Model file for the job. Use its own axes, mm. A direction names the side the tool comes from. Give positions to 0.01 mm unless a question says otherwise; leave off trailing zeros. Write each loop counter-clockwise with the first axis right and the second up, starting at its lowest first coordinate (ties: lowest second). Pieces come first, ordered by that corner, then holes. Notation, with made-up numbers: (1, -11.5) - (6, -11.5) arc R26 cw to (6, 23.5) - close; hole circle Ø7 at (-37.5, 39.25). An arc over 180 degrees is marked (long way). Use CSV: the item, a comma, the result in double quotes.
Autodesk Inventor part; units mm, degrees
ref_plane "Work Plane1" through (-5.5, 5, -9) normal (0, 0, 1) x (1, 0, 0)
ref_plane "YZ Plane" through (0, 0, 0) normal (1, 0, 0) x (0, 1, 0)
ref_plane "XZ Plane" through (0, 0, 0) normal (0, 1, 0) x (-1, 0, 0)
sketch "Sketch1" plane through (0, 0, 0) normal (0, 1, 0) x (-1, 0, 0)
  line L0 (0, 0) -> (0, -10.6)
  line L1 (0, -10.6) -> (-4.5, -10.6)
  line L2 (-4.5, -10.6) -> (-4.5, -39.4)
  line L3 (-4.5, -39.4) -> (0, -39.4)
  line L4 (0, -39.4) -> (0, -50)
  line L5 (0, -50) -> (10, -50)
  line L6 (10, -50) -> (10, -48)
  line L7 (10, -48) -> (15.5, -48)
  line L8 (15.5, -48) -> (15.5, -40)
  line L9 (15.5, -40) -> (10, -40)
  line L10 (10, -40) -> (10, -10)
  line L11 (10, -10) -> (15.5, -10)
  line L12 (15.5, -10) -> (15.5, -2)
  line L13 (15.5, -2) -> (10, -2)
  line L14 (10, -2) -> (10, 0)
  line L15 (10, 0) -> (0, 0)
  line L16 (10.5, -3) -> (0.5, -3)
  line L17 (0.5, -3) -> (0.5, -9)
  line L18 (0.5, -9) -> (10.5, -9)
  line L19 (10.5, -9) -> (10.5, -3)
  line L20 (10.5, -41) -> (0.5, -41)
  line L21 (0.5, -41) -> (0.5, -47)
  line L22 (0.5, -47) -> (10.5, -47)
  line L23 (10.5, -47) -> (10.5, -41)
  dimension "d0" = 20
  dimension "d1" = 50
  dimension "d2" = 10.6
  dimension "d3" = 10.6
  dimension "d4" = 2
  dimension "d5" = 2
  dimension "d6" = 8
  dimension "d7" = 8
  dimension "d8" = 4.5
  dimension "d9" = 5.5
  dimension "d10" = 5.5
  dimension "d11" = 5.5
  dimension "d12" = 5.5
  dimension "d13" = 10
  dimension "d14" = 6
  dimension "d15" = 5
  dimension "d16" = 3
  dimension "d17" = 10
  dimension "d18" = 6
  dimension "d19" = 3
extrude "Extrusion1" add sketch "Sketch1" along normal blind 5
sketch "Sketch2" plane through (-10.5, 0, -9) normal (0, 0, 1) x (1, 0, 0)
  point P0 (10.5, 0)
ref_plane "Work Plane1" through (-5.5, 5, -9) normal (0, 0, 1) x (1, 0, 0)
sketch "Sketch4" plane through (-5.5, 5, -9) normal (0, 0, 1) x (1, 0, 0)
  line L0 (-5, -5) -> (5, -5)
  line L1 (5, -5) -> (-5, -5)
  line L2 (-5, -5) -> (5, -5)
  line L3 (5, -5) -> (-5, -5)
  line L4 (-4.5, -5) -> (5.5, -5)
  line L5 (-10, -5) -> (-4.5, -5)
  line L6 (-4.5, -5) -> (-10, -5)
  line L7 (-10, -5) -> (-4.5, -5)
  line L8 (-4.5, -5) -> (-10, -5)
  line L9 (5.5, -5) -> (-4.5, -5)
  line L10 (10, -5) -> (5.5, -5)
  line L11 (5.5, -5) -> (10, -5)
  line L12 (-5, 0) -> (5, 0)
  line L13 (5, 0) -> (-5, 0)
  line L14 (-5, 0) -> (5, 0)
  line L15 (5, 0) -> (-5, 0)
  line L16 (5.5, 0) -> (10, 0)
  line L17 (10, 0) -> (5.5, 0)
  line L18 (5.5, 0) -> (-4.5, 0)
  line L19 (-4.5, 0) -> (-10, 0)
  line L20 (-10, 0) -> (-4.5, 0)
  line L21 (-4.5, 0) -> (-10, 0)
  line L22 (-10, 0) -> (-4.5, 0)
  line L23 (-4.5, 0) -> (5.5, 0)
  line L24 (5, -5) -> (5, 0)
  line L25 (-5, -5) -> (-5, 0)
  line L26 (5.5, -5) -> (-4.5, -5)
  line L27 (-5, -5) -> (-5, 0) construction
  line L28 (-5, -5) -> (0, -5) construction
  line L29 (5, -5) -> (5, 0)
  line L30 (5, -5) -> (5, 0) construction
  line L31 (5, -5) -> (10, -5) construction
  line L32 (-5, 0) -> (-5, -5)
  line L33 (0, -5) -> (5, -5)
  line L34 (5, 0) -> (5, -5)
  line L35 (5.5, 0) -> (-4.5, 0)
  line L36 (-5, -5) -> (0, -5)
  line L37 (-5, -5) -> (-1, -5)
  line L38 (-1, -5) -> (-1, -4)
  line L39 (5, -5) -> (1, -5)
  line L40 (1, -5) -> (1, -4)
  line L41 (-5, -5) -> (-5, -4)
  line L42 (-5, -5) -> (-5, 0)
  line L43 (5, -5) -> (5, -4)
  arc A0 (5, 0) -> (1, -4) centre (5, -4) ccw
  arc A1 (-1, -4) -> (-5, 0) centre (-5, -4) ccw
  dimension "d26" = 90
  dimension "d28" = 90
  dimension "d48" = 4
  dimension "d49" = 1
  dimension "d50" = 4
  dimension "d51" = 1
  dimension "d52" = 4
extrude "Extrusion2" add sketch "Sketch4" along normal blind 6 contours L25 A1 L38 L0 | L40 A0 L24 L0
sketch "Sketch6" plane through (-10, 0, -48) normal (0, 0, -1) x (-1, 0, 0)
  circle A0 centre (3, 2.5) radius 1.4
  line L0 (0, 0) -> (5.5, 0)
  line L1 (5.5, 0) -> (5.5, 5)
  line L2 (0, 5) -> (5.5, 5)
  line L3 (0, 0) -> (0, 5)
  point P0 (-10, 0)
  dimension "d34" = 2.5
  dimension "d35" = 2.5
  dimension "d47" = 2.8
extrude "Extrusion4" cut sketch "Sketch6" against normal through all contours A0
sketch "Sketch7" plane through (4.5, 0, -39.4) normal (0, 0, -1) x (-1, 0, 0)
  circle A0 centre (2.5, 2.5) radius 1
  line L0 (0, 5) -> (4.5, 5)
  line L1 (0, 0) -> (0, 5)
  point P0 (4.5, 0)
  dimension "d38" = 2
  dimension "d39" = 2.5
  dimension "d40" = 2.5
extrude "Extrusion5" cut sketch "Sketch7" against normal through all
sketch "Sketch8" plane through (-10, 0, -10) normal (0, 0, -1) x (-1, 0, 0)
  point P0 (-10, 0)
sketch "Sketch12" plane through (-0.5, 0, -41) normal (0, 0, -1) x (-1, 0, 0)
  line L0 (6, 1) -> (6, 0)
  line L1 (4, 0) -> (6, 0)
  line L2 (4, 0) -> (4, 1)
  arc A0 (4, 1) -> (0, 5) centre (0, 1) ccw
  line L3 (10, 5) -> (0, 5)
  arc A1 (10, 5) -> (6, 1) centre (10, 1) ccw
  arc A2 (4, 1) -> (0, 5) centre (0, 1) ccw
  arc A3 (10, 5) -> (6, 1) centre (10, 1) ccw
  line L4 (4, 0) -> (6, 0)
  line L5 (6, 1) -> (6, 0)
  line L6 (6, 0) -> (10, 0)
  line L7 (15, 0) -> (9.5, 0)
  line L8 (10, 5) -> (10, 0)
  line L9 (10, 0) -> (6, 0)
  line L10 (9.5, 0) -> (-0.5, 0)
  line L11 (4, 0) -> (0, 0)
  arc A4 (4, 1) -> (0, 5) centre (0, 1) ccw
  line L12 (0, 0) -> (0, 5)
  line L13 (4, 0) -> (4, 1)
  line L14 (4, 0) -> (4, 1)
  dimension "d54" = 5
extrude "Extrusion6" add sketch "Sketch12" along normal blind 6 contours A1 L8 L6 L0 | L10 L12 A0 L2
fillet "Fillet5" radius 2.5 6 edges at (-15.5, 5, -6) (-15.5, 5, -44) (4.5, 5, -25) (-15.5, 0, -6) (4.5, 0, -25) (-15.5, 0, -44)
sketch "Sketch13" plane through (0, 5, 0) normal (0, 1, 0) x (1, 0, 0)
  line L0 (-10, 0) -> (0, 0)
  line L1 (0, 0) -> (-1, 0)
  line L2 (-1, 0) -> (-1, 10.5)
  line L3 (-1, 10.5) -> (0, 10.5)
  line L4 (0, 10.5) -> (0, 0)
  line L5 (0, 39.4) -> (0, 50)
  line L6 (0, 39.4) -> (-1, 39.4)
  line L7 (-1, 39.4) -> (-1, 50)
  line L8 (-1, 50) -> (0, 50)
  line L9 (0, 50) -> (0, 39.4)
  dimension "d58" = 1
extrude "Extrusion7" cut sketch "Sketch13" against normal through all
sketch "Sketch14" plane through (0, 0, 0) normal (0, -1, 0) x (1, 0, 0)
  point P0 (0, 0)
sketch "Sketch15" plane through (0, 5, 0) normal (0, 1, 0) x (1, 0, 0)
  line L0 (-9.5, 23) -> (-2, 23)
  line L1 (-2, 23) -> (-2, 27)
  line L2 (-2, 27) -> (-9.5, 27)
  line L3 (-9.5, 27) -> (-9.5, 23)
  line L4 (-10, 0) -> (-1, 0)
  line L5 (-1, 39.4) -> (-1, 41)
  point P0 (0, 0)
  dimension "d61" = 4
  dimension "d62" = 7.5
  dimension "d63" = 23
  dimension "d64" = 1
extrude "Extrusion8" add sketch "Sketch15" along normal blind 4
sketch "Sketch17" plane through (-9.5, 5, -23) normal (0, 0, 1) x (1, 0, 0)
  line L0 (8.5, 0) -> (-1, 0)
  line L1 (0, 0) -> (0, 4)
  line L2 (0, 0) -> (0, 4)
  line L3 (0, 4) -> (1, 4)
  line L4 (7.5, 4) -> (0, 4)
  line L5 (1, 4) -> (0, 0)
  line L6 (7.5, 4) -> (7.5, 0)
  line L7 (7.5, 0) -> (7.5, 4)
  line L8 (7.5, 4) -> (6.5, 4)
  line L9 (6.5, 4) -> (7.5, 0)
  point P0 (9.5, -5)
  dimension "d69" = 1
  dimension "d70" = 1
extrude "Extrusion9" cut sketch "Sketch17" against normal through all contours L9 L4 L6 | L1 L3 L5
fillet "Fillet6" radius 2 4 edges at (-9, 7, -23) (-2.5, 7, -23) (-2.5, 7, -27) (-9, 7, -27)
sketch "Sketch18" plane through (0, 0, 0) normal (0, -1, 0) x (1, 0, 0)
  line L0 (0, -10.5) -> (0, -10.6)
  line L1 (0, -10.5) -> (0, -10.6)
  line L2 (0, -10.6) -> (-1, -10.6)
  line L3 (-1, -9) -> (-1, -10.5)
  line L4 (-1, -10.6) -> (-1, -10.5)
  line L5 (-1, -10.5) -> (0, -10.5)
  point P0 (0, 0)
  dimension "d74" = 1
extrude "Extrusion10" cut sketch "Sketch18" against normal through all
properties part number "tracks"
(1) Saw through at B-B, the plane z = -5. Count the separate pieces of the cut face and the enclosed holes in it, then the cut area to 3 significant figures.
Checked values:
separate pieces,"2"
enclosed holes,"1"
area,"46.8 mm^2"
(2) Flat gauge pins, fed straight in: P1, Ø1.5, axis at x = 1.5, y = 3, coming from the -Z side; P2, Ø1.6, axis at y = 3, z = -49, coming from the -X side; P3, Ø8, axis at x = -4, z = -36.5, coming from the +Y side. Where does each tip first touch, or does it go through?
Checked values:
P1,"stops at z = -39.4"
P2,"stops at x = -10"
P3,"stops at y = 5"
(3) 3-axis set-ups, long thin cutter, end or side, ignore diameter. For faces 4 (the face through (-6.5, 0.5, -44)), 5 (the face through (-6, 7, -23)), 6 (the face through (-7.641, 3.797, -43.958)): which of +Z, -Z, +X, -X, +Y, -Y reach the whole face in a straight line?
Checked values:
face 4,"+Y, -Y"
face 5,"+Z, +X, -X, +Y"
face 6,"+Y"
(4) Saw through at A-A, the plane x = -11. List the corners of the cut face in (y, z), then the cut area to 3 significant figures.
Checked values:
outline,"(0, -48) - (5, -48) - (5, -40) - (0, -40) - close; (0, -10) - (5, -10) - (5, -2) - (0, -2) - close"
area,"80.0 mm^2"
(5) Saw through at D-D, the plane x = -5.75. List the corners of the cut face in (y, z), then the cut area to 3 significant figures.
Checked values:
outline,"(0, -50) - (5, -50) - (5, -47) - (0, -47) - close; (0, -41) - (5, -41) - (5, -27) - (9, -27) - (9, -23) - (5, -23) - (5, -9) - (0, -9) - close; (0, -3) - (5, -3) - (5, 0) - (0, 0) - close"
area,"206 mm^2"
(6) Wall check: probe 1 along Y at (x, z) = (2, -27); probe 2 along Z at (x, y) = (-14.5, 1.75); probe 3 along X at (y, z) = (1.5, -43). Give the ranges that are in metal, low to high. Write a range as [from, to].
Checked values:
probe 1,"y = [0, 1.5], [3.5, 5]"
probe 2,"z = [-48, -40], [-10, -2]"
probe 3,"x = [-15.29, -13.98], [-12.02, -6.53], [-4.47, -1]"
(7) Pull direction Z, two halves, no side cores. Call faces 1 (the face through (-10, 2, -25)), 2 (the face through (-1, 3, -45)), 3 (the face through (-3.106, 7.073, -23.601)): released by +Z, released by -Z, zero draft, split by the parting line, or undercut.
Checked values:
face 1,"undercut"
face 2,"zero draft"
face 3,"released by +Z"
